The listing builds one solid part. Answer for the finished solid, in the listing's coordinates (mm). A direction names the side the tool comes from. Give positions to 0.01 mm unless a question says otherwise; leave off trailing zeros. Loops run counter-clockwise (first coordinate to the right, second up) from the corner with the lowest first, then second, coordinate; pieces in that order, holes last. Notation, with made-up numbers: (-25, 48.5) - (-20, 48.5) arc R13 cw to (-20, 57.5) - close; hole circle Ø3 at (24, 44.5). An arc over 180 degrees is marked (long way). Write item = value, one per line. Start each with the question number.
1) The part is cut by section B-B on z = 2. State how many separate pieces and enclosed holes the cut face has, plus the area to 3 significant figures.
2) The part is cut by section A-A on x = 28. Write down the section's boundary in (y, z), plus the area to 3 significant figures.
3) Consider probe 1 along Z at (x, y) = (17, 3); probe 2 along X at (y, z) = (19, -4.5); probe 3 along Y at (x, z) = (38, 0.75). Determine where each line is inside the solid, lowest interval first.
4) The part is cut by section C-C on x = -53.5. Write down the section's boundary in (y, z), plus the area to 3 significant figures.
5) The mould has two halves that part along Y. Classify faces 6 (the flat face through (18, 5, -24)), 7 (the flat face through (31, -12.5, 0)), 8 (the cylindrical face through (13.364, 3.235, 25.8)): +Y half, -Y half, draft (parallel to the pull), parting line (faces both ways), or undercut.
6) Flat-ended cylindrical pins translate along their axes: P1, Ø10, axis at y = 9.5, z = 7.5, coming from the -X side; P2, Ø3, axis at x = -29, y = -21, coming from the +Z side; P3, Ø5, axis at x = -37.5, y = 3.5, coming from the +Z side. Find the tip coordinate at first contact, or state that the pin passes through.
7) Which of the six approach directions +Z, -Z, +X, -X, +Y, -Y give full straight-line access (tool end or side, diameter ignored) to faces 1 (the cylindrical face through (-66.214, 17.042, -1.951)), 2 (the flat face through (33, 20, -5)), 3 (the flat face through (-39, 10, 16)), 4 (the flat face through (35, 20, 5)), 5 (the flat face through (12, 5, 27))?
from build123d import *

# Parameters (mm, degrees)
SKETCH3_R                                      = 20
CUT_EXTRUDE1_DEPTH                             = 20
CUT_EXTRUDE2_START                             = -20
SKETCH4_R                                      = 20
CUT_EXTRUDE2_DEPTH                             = 20
SKETCH5_R                                      = 15
CUT_EXTRUDE3_DEPTH                             = 20
CHAMFER1_SIZE                                  = 2
CHAMFER2_SIZE                                  = 2
BOSS_EXTRUDE1_DEPTH                            = 5
CSK_FOR_M4_FLAT_HEAD_MACHINE_SCREW1_AT_2_COUNT = 2
CSK_FOR_M4_FLAT_HEAD_MACHINE_SCREW1_AT_2_PITCH = 40
BOSS_EXTRUDE2_DEPTH                            = 5
CBORE_FOR_M5_HEX_HEAD_BOLT1_AT_2_COUNT         = 2
CBORE_FOR_M5_HEX_HEAD_BOLT1_AT_2_PITCH         = 60.621778265
BOSS_EXTRUDE3_DEPTH                            = 20
CUT_EXTRUDE4_DEPTH                             = 20
CUT_EXTRUDE5_DEPTH                             = 10
CUT_EXTRUDE6_START                             = -10
CUT_EXTRUDE6_DEPTH                             = 10
FILLET1_R                                      = 5


with BuildPart() as part:
    # Sketch1 → Revolve1 (revolve)
    with BuildSketch(Plane.XY):
        Polygon((0, 0), (0, 30), (-25, 30), (-25, -30), (0, -30), align=None)
    revolve(axis=Axis((0, 0, 0), (0, -1, 0)))

    # Sketch3 → Cut-Extrude1 (cut)
    with BuildSketch(Plane(origin=(0, 30, 0), x_dir=(1, 0, 0), z_dir=(0, 1, 0))):
        with Locations(Location((0, 0, 0), (0, 0, 180))):
            Circle(SKETCH3_R)
    extrude(amount=-CUT_EXTRUDE1_DEPTH, mode=Mode.SUBTRACT)

    # Sketch4 → Cut-Extrude2 (cut)
    with BuildSketch(Plane.XZ.offset(30).offset(CUT_EXTRUDE2_START)):
        with Locations(Location((0, 0, 0), (0, 0, 180))):
            Circle(SKETCH4_R)
    extrude(amount=CUT_EXTRUDE2_DEPTH, mode=Mode.SUBTRACT)

    # Sketch5 → Cut-Extrude3 (cut)
    with BuildSketch(Plane(origin=(0, 10, 0), x_dir=(1, 0, 0), z_dir=(0, 1, 0))):
        with Locations(Location((0, 0, 0), (0, 0, 180))):
            Circle(SKETCH5_R)
    extrude(amount=-CUT_EXTRUDE3_DEPTH, mode=Mode.SUBTRACT)

    # Chamfer1
    chamfer1_edges = [part.edges().sort_by_distance(p)[0] for p in [
        (20, -30, 0),
    ]]
    chamfer(chamfer1_edges, length=CHAMFER1_SIZE)

    # Chamfer2
    chamfer2_edges = [part.edges().sort_by_distance(p)[0] for p in [
        (20, 30, 0),
    ]]
    chamfer(chamfer2_edges, length=CHAMFER2_SIZE)

    # Sketch10 → Boss-Extrude1 (add, symmetric)
    with BuildSketch(Plane.XY):
        with BuildLine():
            Line((25, 27.5), (23, 27.5))
            Line((23, 27.5), (23, 12.5))
            Line((23, 12.5), (38, 12.5))
            ThreePointArc((38, 12.5), (45.5, 20), (38, 27.5))
            Line((38, 27.5), (25, 27.5))
        make_face()
        with BuildLine():
            Line((23, -12.5), (38, -12.5))
            ThreePointArc((38, -12.5), (45.5, -20), (38, -27.5))
            Line((38, -27.5), (25, -27.5))
            Line((25, -27.5), (23, -27.5))
            Line((23, -27.5), (23, -12.5))
        make_face()
    extrude(amount=BOSS_EXTRUDE1_DEPTH, both=True)

    # Sketch12 → CSK for M4 Flat Head Machine Screw1 (revolve, cut)
    with BuildSketch(Plane(origin=(38, 20, -5), x_dir=(0, 1, 0), z_dir=(1, 0, 0))):
        Polygon((0, 0), (0, 30), (2.25, 30), (2.25, 2.45), (4.7, 0), align=None)
    csk_for_m4_flat_head_machine_screw1 = revolve(axis=Axis((38, 20, -11.35), (0, 0, 1)), mode=Mode.SUBTRACT)

    # CSK for M4 Flat Head Machine Screw1 at 2: CSK for M4 Flat Head Machine Screw1 ×2
    with Locations(*[(0, -i * CSK_FOR_M4_FLAT_HEAD_MACHINE_SCREW1_AT_2_PITCH, 0) for i in range(1, CSK_FOR_M4_FLAT_HEAD_MACHINE_SCREW1_AT_2_COUNT)]):
        add(csk_for_m4_flat_head_machine_screw1, mode=Mode.SUBTRACT)

    # Sketch13 → Boss-Extrude2 (add, symmetric)
    with BuildSketch(Plane(origin=(0, 0, 0), x_dir=(1, 0, 0), z_dir=(0, 1, 0))):
        with BuildLine():
            Line((9.705771366, 34.810889132), (3.867675156, 24.699009877))
            ThreePointArc((3.867675156, 24.699009877), (12.5, 21.650635095), (19.456132424, 15.699009877))
            Line((19.456132424, 15.699009877), (25.294228634, 25.810889132))
            ThreePointArc((25.294228634, 25.810889132), (22, 38.105117767), (9.705771366, 34.810889132))
        make_face()
        with BuildLine():
            Line((9.705771366, -34.810889132), (3.867675156, -24.699009877))
            ThreePointArc((3.867675156, -24.699009877), (12.5, -21.650635095), (19.456132424, -15.699009877))
            Line((19.456132424, -15.699009877), (25.294228634, -25.810889132))
            ThreePointArc((25.294228634, -25.810889132), (22, -38.105117767), (9.705771366, -34.810889132))
        make_face()
    extrude(amount=BOSS_EXTRUDE2_DEPTH, both=True)

    # Sketch15 → CBORE for M5 Hex Head Bolt1 (revolve, cut)
    with BuildSketch(Plane(origin=(17.5, 5, -30.310889132), x_dir=(0, 0, 1), z_dir=(1, 0, 0))):
        Polygon((0, 0), (0, 35), (2.75, 35), (2.75, 3.58), (6.12, 3.58), (6.12, 0), align=None)
    cbore_for_m5_hex_head_bolt1 = revolve(axis=Axis((17.5, 11.35, -30.310889132), (0, -1, 0)), mode=Mode.SUBTRACT)

    # CBORE for M5 Hex Head Bolt1 at 2: CBORE for M5 Hex Head Bolt1 ×2
    with Locations(*[(0, 0, i * CBORE_FOR_M5_HEX_HEAD_BOLT1_AT_2_PITCH) for i in range(1, CBORE_FOR_M5_HEX_HEAD_BOLT1_AT_2_COUNT)]):
        add(cbore_for_m5_hex_head_bolt1, mode=Mode.SUBTRACT)



with BuildPart() as body_2:
    # Sketch2 → Revolve2 (revolve)
    with BuildSketch(Plane.XY, mode=Mode.PRIVATE) as revolve2_sk:
        Polygon((-75, 0), (-75, 20), (-87.5, 20), (-87.5, -20), (-75, -20), align=None)
    revolve(revolve2_sk.sketch.rotate(Axis((-75, 0, 0), (0, 1, 0)), 270), axis=Axis((-75, 0, 0), (0, 1, 0)))

    # Sketch9 → CBORE for M8 Pan Head Machine Screw2 (revolve, cut)
    with BuildSketch(Plane(origin=(-75, 20, 0), x_dir=(0, 0, 1), z_dir=(1, 0, 0))):
        Polygon((0, 0), (0, 50), (4.5, 50), (4.5, 6), (9, 6), (9, 0), align=None)
    revolve(axis=Axis((-75, 26.35, 0), (0, -1, 0)), mode=Mode.SUBTRACT)


with BuildPart() as part_1:
    add(part.part)

    add(body_2.part)  # Boss-Extrude3 merges body 2
    # Sketch16 → Boss-Extrude3 (add, symmetric)
    with BuildSketch(Plane(origin=(0, 0, 0), x_dir=(1, 0, 0), z_dir=(0, 1, 0))):
        with BuildLine():
            Line((-75, 12.5), (-8.11, 23.647999915))
            ThreePointArc((-8.11, 23.647999915), (-25, 0), (-8.11, -23.647999915))
            Line((-8.11, -23.647999915), (-75, -12.5))
            ThreePointArc((-75, -12.5), (-62.5, 0), (-75, 12.5))
        make_face()
    extrude(amount=BOSS_EXTRUDE3_DEPTH, both=True)

    # Sketch17 → Cut-Extrude4 (cut, symmetric)
    with BuildSketch(Plane(origin=(0, 0, 0), x_dir=(1, 0, 0), z_dir=(0, 1, 0))):
        with BuildLine():
            Line((-34.581559949, -14.167240529), (-61.524552888, -9.676876005))
            ThreePointArc((-61.524552888, -9.676876005), (-63.694159972, -8.0995569), (-63.73497603, -5.41749342))
            ThreePointArc((-63.73497603, -5.41749342), (-62.5, 0), (-63.73497603, 5.41749342))
            ThreePointArc((-63.73497603, 5.41749342), (-63.694159972, 8.0995569), (-61.524552888, 9.676876005))
            Line((-61.524552888, 9.676876005), (-34.581559949, 14.167240529))
            ThreePointArc((-34.581559949, 14.167240529), (-30.048614002, 12.586186956), (-28.936790513, 7.915943077))
            ThreePointArc((-28.936790513, 7.915943077), (-30, 0), (-28.936790513, -7.915943077))
            ThreePointArc((-28.936790513, -7.915943077), (-30.048614002, -12.586186956), (-34.581559949, -14.167240529))
        make_face()
    extrude(amount=CUT_EXTRUDE4_DEPTH, both=True, mode=Mode.SUBTRACT)

    # Sketch18 → Cut-Extrude5 (cut)
    with BuildSketch(Plane(origin=(0, 20, 0), x_dir=(1, 0, 0), z_dir=(0, 1, 0))):
        with BuildLine():
            Line((-30, 0), (-25, 0))
            ThreePointArc((-25, 0), (-20.34391801, -14.530141087), (-8.11, -23.647999915))
            Line((-8.11, -23.647999915), (-75, -12.5))
            ThreePointArc((-75, -12.5), (-68.346755219, -10.582265064), (-63.73497603, -5.41749342))
            ThreePointArc((-63.73497603, -5.41749342), (-63.694159972, -8.0995569), (-61.524552888, -9.676876005))
            Line((-61.524552888, -9.676876005), (-34.581559949, -14.167240529))
            ThreePointArc((-34.581559949, -14.167240529), (-30.048614002, -12.586186956), (-28.936790513, -7.915943077))
            ThreePointArc((-28.936790513, -7.915943077), (-29.733009563, -3.993512527), (-30, 0))
        make_face()
    extrude(amount=-CUT_EXTRUDE5_DEPTH, mode=Mode.SUBTRACT)

    # Sketch19 → Cut-Extrude6 (cut)
    with BuildSketch(Plane.XZ.offset(20).offset(CUT_EXTRUDE6_START)):
        with BuildLine():
            Line((-30, 0), (-25, 0))
            ThreePointArc((-25, 0), (-20.34391801, -14.530141087), (-8.11, -23.647999915))
            Line((-8.11, -23.647999915), (-75, -12.5))
            ThreePointArc((-75, -12.5), (-68.346755219, -10.582265064), (-63.73497603, -5.41749342))
            ThreePointArc((-63.73497603, -5.41749342), (-63.611614037, -8.056719366), (-61.524552888, -9.676876005))
            Line((-61.524552888, -9.676876005), (-33.759588932, -14.235266923))
            ThreePointArc((-33.759588932, -14.235266923), (-29.784880186, -12.268695739), (-28.936790513, -7.915943077))
            ThreePointArc((-28.936790513, -7.915943077), (-29.733009563, -3.993512527), (-30, 0))
        make_face()
    extrude(amount=CUT_EXTRUDE6_DEPTH, mode=Mode.SUBTRACT)

    # Fillet1
    # the kernel refuses this fillet: 5 mm, written as the material it adds along each edge
    with BuildSketch(Plane(origin=(-42.5, 10, 0), x_dir=(0, 0, 1), z_dir=(1, 0, 0))) as fillet1_piece_1_section:
        with BuildLine():
            CenterArc((FILLET1_R, -FILLET1_R), FILLET1_R, 90, 90)
            Line((0, -FILLET1_R), (0, 0))
            Line((0, 0), (FILLET1_R, 0))
        make_face()
    fillet1_piece_1 = extrude(amount=30, mode=Mode.PRIVATE)
    fillet1_piece_1 = fillet1_piece_1 & Plane(origin=(0, 11.115866263, 0), x_dir=(-0.9645596837736771, 0, -0.26386476922549573), z_dir=(0, 1, 0)) * Cylinder(30, 80, mode=Mode.PRIVATE)
    fillet1_piece_1 = fillet1_piece_1 - Plane(origin=(0, 11.115866263, 0), x_dir=(-1, 0, 0), z_dir=(0, 1, 0)) * Cylinder(20, 80, mode=Mode.PRIVATE)
    add(fillet1_piece_1)
    with BuildSketch(Plane(origin=(-42.5, -10, 0), x_dir=(0, 0, -1), z_dir=(1, 0, 0))) as fillet1_piece_2_section:
        with BuildLine():
            CenterArc((FILLET1_R, -FILLET1_R), FILLET1_R, 90, 90)
            Line((0, -FILLET1_R), (0, 0))
            Line((0, 0), (FILLET1_R, 0))
        make_face()
    fillet1_piece_2 = extrude(amount=30, mode=Mode.PRIVATE)
    fillet1_piece_2 = fillet1_piece_2 & Plane(origin=(0, -11.11586543, 0), x_dir=(-0.9645596837736771, 0, -0.26386476922549573), z_dir=(0, 1, 0)) * Cylinder(30, 80, mode=Mode.PRIVATE)
    fillet1_piece_2 = fillet1_piece_2 - Plane(origin=(0, -11.11586543, 0), x_dir=(-1, 0, 0), z_dir=(0, 1, 0)) * Cylinder(20, 80, mode=Mode.PRIVATE)
    add(fillet1_piece_2)
    # the kernel refuses this fillet: 5 mm, written as the material it takes off along each edge
    with BuildSketch(Plane(origin=(-42.5, 20, 0), x_dir=(0, -1, 0), z_dir=(1, 0, 0))) as fillet1_2_piece_1_section:
        with BuildLine():
            CenterArc((FILLET1_R, FILLET1_R), FILLET1_R, 180, 90)
            Line((0, FILLET1_R), (0, 0))
            Line((0, 0), (FILLET1_R, 0))
        make_face()
    fillet1_2_piece_1 = extrude(amount=30, mode=Mode.PRIVATE)
    fillet1_2_piece_1 = fillet1_2_piece_1 - Plane(origin=(0, 18.884144213, 0), x_dir=(-1, 0, 0), z_dir=(0, -1, 0)) * Cylinder(25, 80, mode=Mode.PRIVATE)
    add(fillet1_2_piece_1, mode=Mode.SUBTRACT)
    with BuildSketch(Plane(origin=(-42.5, -20, 0), x_dir=(0, 0, 1), z_dir=(1, 0, 0))) as fillet1_2_piece_2_section:
        with BuildLine():
            CenterArc((FILLET1_R, -FILLET1_R), FILLET1_R, 90, 90)
            Line((0, -FILLET1_R), (0, 0))
            Line((0, 0), (FILLET1_R, 0))
        make_face()
    fillet1_2_piece_2 = extrude(amount=30, mode=Mode.PRIVATE)
    fillet1_2_piece_2 = fillet1_2_piece_2 - Plane(origin=(0, -18.884130023, 0), x_dir=(-1, 0, 0), z_dir=(0, -1, 0)) * Cylinder(25, 80, mode=Mode.PRIVATE)
    add(fillet1_2_piece_2, mode=Mode.SUBTRACT)


solid = part_1.part
Answer below:
q1.separate_pieces = 4
q1.enclosed_holes = 2
q1.area = 2,090 mm2
q2.outline = (-27.5, -5) - (-12.5, -5) - (-12.5, 5) - (-27.5, 5) - close; (12.5, -5) - (27.5, -5) - (27.5, 5) - (12.5, 5) - close
q2.area = 300 mm2
q3.probe_1 = -39.3 to -36.41, -24.21 to 24.21, 36.41 to 39.3
q3.probe_2 = -86.66 to -82.79, -67.21 to -63.34, -29.66 to -19.49, 19.49 to 33.92, 42.08 to 45.43
q3.probe_3 = -27.5 to -22.25, -17.75 to -12.5, 12.5 to 17.75, 22.25 to 27.5
q4.outline = (-20, 11.01) - (10, 11.01) - (10, 16.08) - (-20, 16.08) - close; (-10, -16.08) - (20, -16.08) - (20, -11.01) - (-10, -11.01) - close
q4.area = 304 mm2
q5.face_6 = +Y half
q5.face_7 = undercut
q5.face_8 = draft
q6.P1 = -87.25
q6.P2 = 20.35
q6.P3 = 19.17
q7.face_1 = +Y
q7.face_2 = -Z, +X, +Y, -Y
q7.face_3 = +Z, +Y
q7.face_4 = +Z, +X, +Y, -Y
q7.face_5 = +Z, +X, +Y
